```python
from build123d import *

# Parameters (mm, degrees)
BOSS_EXTRUDE1_DEPTH = 100


with BuildPart() as part:
    # Sketch1 → Boss-Extrude1 (new body)
    with BuildSketch(Plane(origin=(32.364284334, 0, 0), x_dir=(0, 0, -1), z_dir=(1, 0, 0))):
        with BuildLine():
            ThreePointArc((-10.800866483, 33.955059464), (-10.773935743, 33.156778763), (-10.014083429, 33.402953098))
            ThreePointArc((-10.014083429, 33.402953098), (-7.875866483, 34.92701851), (-5.737649536, 33.402953098))
            ThreePointArc((-5.737649536, 33.402953098), (-4.977797222, 33.156778763), (-4.950866483, 33.955059464))
            Line((-4.950866483, 33.955059464), (-4.950866483, 34.079201599))
            Line((-4.950866483, 34.079201599), (-3.496394261, 35.533673821))
            Line((-3.496394261, 35.533673821), (-12.255338704, 35.533673821))
            Line((-12.255338704, 35.533673821), (-10.800866483, 34.079201599))
            Line((-10.800866483, 34.079201599), (-10.800866483, 33.955059464))
        make_face()
    extrude(amount=BOSS_EXTRUDE1_DEPTH)


solid = part.part
```
Source: CAD feature listing. Evaluate the final solid. Frame: model axes, mm. Coordinates: 2 decimals unless noted, no trailing zeros. Loops run counter-clockwise (first coordinate to the right, second up) from the corner with the lowest first, then second, coordinate; pieces in that order, holes last. Notation, with made-up numbers: (-31.75, -1.75) - (2.25, -1.75) arc R8 cw to (2.25, 4.25) - close; hole circle Ø7 at (-26.5, -16.5). An arc over 180 degrees is marked (long way). Answer as CSV lines item,"result".
1. Section B-B (z = 9). Return loops of the section in (x, y).
Established:
outline,"(32.36, 34.63) - (132.36, 34.63) - (132.36, 35.53) - (32.36, 35.53) - close"
2. Section A-A (x = 46). Return loops of the section in (y, z) (3 decimals), then the cut area to 3 significant figures.
Established:
outline,"(33.403, 5.738) arc R0.5 ccw (long way) to (33.955, 4.951) - (34.079, 4.951) - (35.534, 3.496) - (35.534, 12.255) - (34.079, 10.801) - (33.955, 10.801) arc R0.5 ccw (long way) to (33.403, 10.014) arc R2.262 cw to start"
area,"10.4 mm2"
3. Ray query, line 1 (Z direction, x = 42.5, y = 34.2); line 2 (Z direction, x = 83, y = 33.2); line 3 (Z direction, x = 117.5, y = 35.4). Return the intervals inside material, ascending.
Established:
line 1,"z = 4.83 to 6.21, 9.54 to 10.92"
line 2,"z = 4.92 to 5.61, 10.15 to 10.83"
line 3,"z = 3.63 to 12.12"
